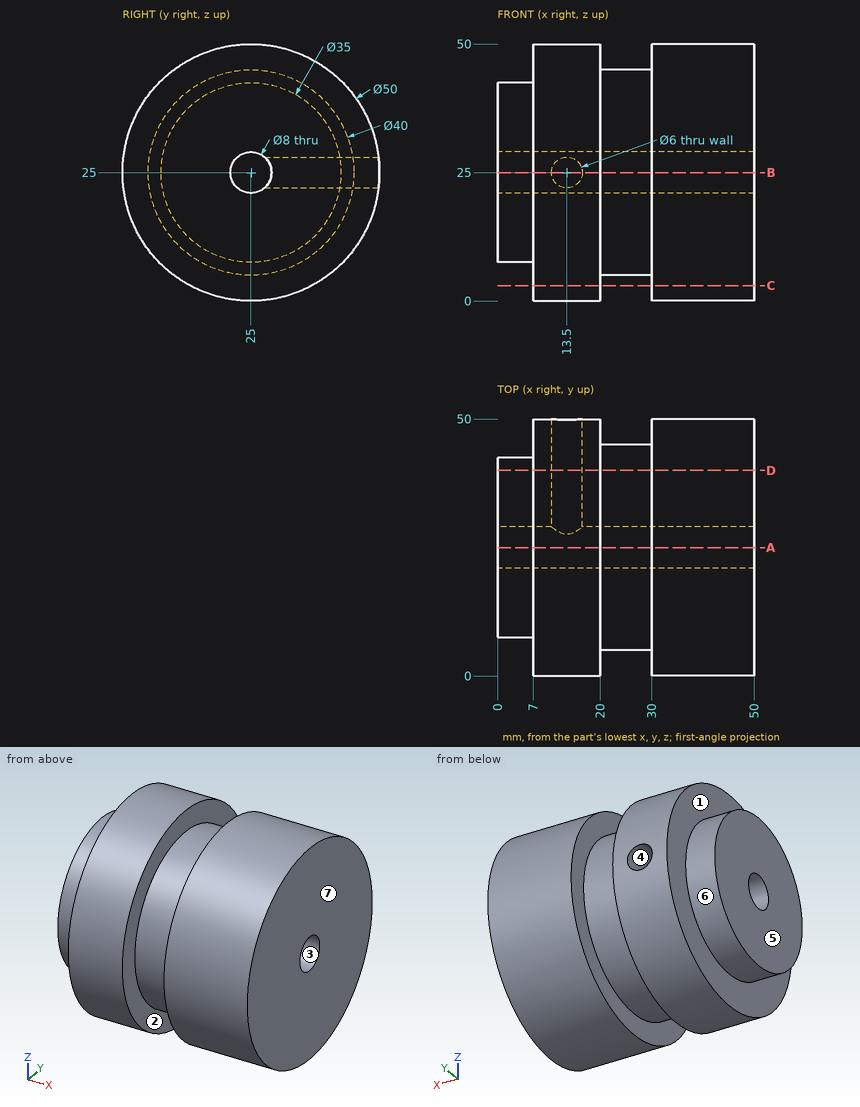
Input: dimensioned drawing with shaded views. Units: mm. Origin: part minimum x, y, z. A direction names the side the tool comes from. Coordinates: 2 decimals unless noted, no trailing zeros. Order: outer loops, then holes, each group sorted by start corner. A loop starts at its lowest first (then second) coordinate and runs counter-clockwise, first axis right, second up. Notation, with made-up numbers: (-40, -3.5) - (-6, -3.5) arc R13 cw to (-6, 5.5) - close; hole circle Ø7 at (-13, -8). An arc over 180 degrees is marked (long way). Return JSON: item names as keys, results as strings. Group by question number.
1. Cut plane A-A (y = 25). Output: boundary loops of the cut face in (x, z).
2. Cut plane B-B (z = 25). Output: boundary loops of the cut face in (x, y).
3. Material intervals for line 1 along Z through (x, y) = (35, 25); line 2 along X through (y, z) = (7.5, 40); line 3 along X through (y, z) = (10.5, 13.5), sorted ascending. Write a range as [from, to].
4. Cut plane D-D (y = 40). Output: boundary loops of the cut face in (x, z), plus the area to 3 significant figures.
5. Set-up query: the marked faces 1, 2 and 3. Return all of +Z, -Z, +X, -X, +Y, -Y with unobstructed straight access to the full face (end or side cutting, diameter ignored); none if empty.
6. Pin query (flat end, axial travel): pin 1 (6 mm diameter, centred on x = 21.5, z = 8, fed in from -Y); pin 2 (3 mm diameter, centred on y = 11.5, z = 42, fed in from -X); pin 3 (1 mm diameter, centred on x = 31, y = 28, fed in from +Z). Return the tip coordinate at first contact, or that it passes through.
7. Pull-direction query (X, two-part tool) for the marked faces 4, 5, 6 and 7; classes: pulls with the +X half, pulls with the -X half, needs draft (parallel to the pull), parting line crosses it, or undercut.
8. Cut plane C-C (z = 3). Output: boundary loops of the cut face in (x, y).
Resolved:
{
 "1": {"outline": "(0, 7.5) - (7, 7.5) - (7, 0) - (20, 0) - (20, 5) - (30, 5) - (30, 0) - (50, 0) - (50, 21) - (0, 21) - close; (0, 29) - (50, 29) - (50, 50) - (30, 50) - (30, 45) - (20, 45) - (20, 50) - (7, 50) - (7, 42.5) - (0, 42.5) - close"},
 "2": {"outline": "(0, 7.5) - (7, 7.5) - (7, 0) - (20, 0) - (20, 5) - (30, 5) - (30, 0) - (50, 0) - (50, 21) - (0, 21) - close; (0, 29) - (10.5, 29) - (10.5, 50) - (7, 50) - (7, 42.5) - (0, 42.5) - close; (16.5, 29) - (50, 29) - (50, 50) - (30, 50) - (30, 45) - (20, 45) - (20, 50) - (16.5, 50) - close"},
 "3": {"line 1": "z = [0, 21], [29, 50]", "line 2": "x = [7, 20], [30, 50]", "line 3": "x = [7, 50]"},
 "4": {"outline": "(0, 15.99) - (7, 15.99) - (7, 5) - (20, 5) - (20, 11.77) - (30, 11.77) - (30, 5) - (50, 5) - (50, 45) - (30, 45) - (30, 38.23) - (20, 38.23) - (20, 45) - (7, 45) - (7, 34.01) - (0, 34.01) - close; hole circle Ø6 at (13.5, 25)", "area": "1,680 mm²"},
 "5": {"face 1": "-X", "face 2": "none", "face 3": "+X, -X"},
 "6": {"pin 1": "stops at y = 4.57", "pin 2": "stops at x = 7", "pin 3": "stops at z = 49.87"},
 "7": {"face 4": "undercut", "face 5": "pulls with the -X half", "face 6": "needs draft", "face 7": "pulls with the +X half"},
 "8": {"outline": "(7, 13.13) - (20, 13.13) - (20, 36.87) - (7, 36.87) - close; (30, 13.13) - (50, 13.13) - (50, 36.87) - (30, 36.87) - close"}
}
